Could you check a few things on this model? Use its own coordinates, in mm. A direction names the side the tool comes from. Round coordinates to 2 decimals unless told otherwise and drop trailing zeros. Write each loop counter-clockwise with the first axis right and the second up, starting at its lowest first coordinate (ties: lowest second). Pieces come first, ordered by that corner, then holes. Notation, with made-up numbers: (-14, 67.5) -> (38, 67.5) arc R37 cw to (38, 105.5) -> close; hole circle Ø9 at (70, -34). An arc over 180 degrees is marked (long way). One line per question, with ' | ' between items. Start each with the question number.
1. Imagine slicing it at D-D, the plane y = 33.5. List the corners of the cut face in (x, z) for me.
2. For faces 5 (the flat face through (56.91, -29.28, 0.49)), 6 (the flat face through (-60, -62, 1)), which set-ups out of +Z, -Z, +X, -X, +Y, -Y let a thin tool reach every point of the face, with its end or its side?
3. Imagine slicing it at A-A, the plane y = -37.5. List the corners of the cut face in (x, z) for me, and give its area (3 significant figures).
4. Imagine slicing it at B-B, the plane x = 22. List the corners of the cut face in (y, z) for me, and give its area (3 significant figures).
5. If I drill on line 1 along Y through (x, z) = (52.5, 12.5); line 2 along X through (y, z) = (-51, 13.25); line 3 along Y through (x, z) = (2, 9.25), over which ranges is the centre line in solid material (lowest first)? Write a range as [from, to].
6. Imagine slicing it at C-C, the plane z = 11.25. State how many separate pieces and enclosed holes the cut face has, and give its area (3 significant figures).
7. Thinking about a two-plate mould opening in Y: for faces 1 (the flat face through (-1, 68.5, 12)), 2 (the flat face through (-65.5, -1, 12)), 3 (the flat face through (-63.5, 44, 12)), 4 (the flat face through (32, -66, 12)), which applies, released by +Y, released by -Y, zero draft, split by the parting line, or undercut?
8. For pin 1 Ø6.5 at (x, y) = (59, -17.5) entering from +Z, with a flat end and sliding along its axis, tell me the tip position at first contact or that it passes through.
from build123d import *

# Parameters (mm, degrees)
F0_W     = 131
F0_H     = 137
F1_DEPTH = 24
F2_DEPTH = 1
F3_R     = 2


with BuildPart() as f1:
    # F0 (on Top) → F1 (new body)
    with BuildSketch(Plane.XY):
        Rectangle(F0_W, F0_H)
        Polygon((63.5, -53.262113756), (63.5, -66), (50.5, -66), (13.5, -66), (0.5, -66), (-0.5, -66), (-13.5, -66), (-50.5, -66), (-63.5, -66), (-63.5, -53.262113756), (-63.5, -35.737886244), (-63.5, -23), (-63.5, -21.5), (-63.5, -8.762113756), (-63.5, 8.762113756), (-63.5, 21.5), (-63.5, 23), (-63.5, 35.737886244), (-63.5, 53.262113756), (-63.5, 66), (-50.5, 66), (-13.5, 66), (-0.5, 66), (0.5, 66), (13.5, 66), (50.5, 66), (63.5, 66), (63.5, 53.262113756), (63.5, 35.737886244), (63.5, 23), (63.5, 21.5), (63.5, 8.762113756), (63.5, -8.762113756), (63.5, -21.5), (63.5, -23), (63.5, -35.737886244), align=None, mode=Mode.SUBTRACT)
        Polygon((-0.5, -66), (0.5, -66), (0.5, -53.262113756), (0.5, -35.737886244), (0.5, -23), (0.5, -21.5), (0.5, -8.762113756), (0.5, 8.762113756), (0.5, 21.5), (0.5, 23), (0.5, 35.737886244), (0.5, 53.262113756), (0.5, 66), (-0.5, 66), (-0.5, 53.262113756), (-0.5, 35.737886244), (-0.5, 23), (-0.5, 21.5), (-0.5, 8.762113756), (-0.5, -8.762113756), (-0.5, -21.5), (-0.5, -23), (-0.5, -35.737886244), (-0.5, -53.262113756), align=None)
        Polygon((50.5, 21.5), (63.5, 21.5), (63.5, 23), (50.5, 23), (13.5, 23), (0.5, 23), (0.5, 21.5), (13.5, 21.5), align=None)
        Polygon((-13.5, 21.5), (-0.5, 21.5), (-0.5, 23), (-13.5, 23), (-50.5, 23), (-63.5, 23), (-63.5, 21.5), (-50.5, 21.5), align=None)
        Polygon((-13.5, -23), (-0.5, -23), (-0.5, -21.5), (-13.5, -21.5), (-50.5, -21.5), (-63.5, -21.5), (-63.5, -23), (-50.5, -23), align=None)
        Polygon((50.5, -23), (63.5, -23), (63.5, -21.5), (50.5, -21.5), (13.5, -21.5), (0.5, -21.5), (0.5, -23), (13.5, -23), align=None)
    extrude(amount=F1_DEPTH)

    # F0 (on Top) → F2 (join)
    with BuildSketch(Plane.XY):
        Polygon((-63.5, 66), (-63.5, 53.262113756), (-50.5, 66), align=None)
        Polygon((-63.5, 35.737886244), (-63.5, 23), (-50.5, 23), align=None)
        Polygon((-13.5, 66), (-0.5, 53.262113756), (-0.5, 66), align=None)
        Polygon((-13.5, 23), (-0.5, 23), (-0.5, 35.737886244), align=None)
        Polygon((0.5, 66), (0.5, 53.262113756), (13.5, 66), align=None)
        Polygon((50.5, 66), (63.5, 53.262113756), (63.5, 66), align=None)
        Polygon((50.5, 23), (63.5, 23), (63.5, 35.737886244), align=None)
        Polygon((0.5, 35.737886244), (0.5, 23), (13.5, 23), align=None)
        Polygon((0.5, 21.5), (0.5, 8.762113756), (13.5, 21.5), align=None)
        Polygon((-13.5, 21.5), (-0.5, 8.762113756), (-0.5, 21.5), align=None)
        Polygon((-63.5, 21.5), (-63.5, 8.762113756), (-50.5, 21.5), align=None)
        Polygon((-63.5, -8.762113756), (-63.5, -21.5), (-50.5, -21.5), align=None)
        Polygon((-13.5, -21.5), (-0.5, -21.5), (-0.5, -8.762113756), align=None)
        Polygon((50.5, -21.5), (63.5, -21.5), (63.5, -8.762113756), align=None)
        Polygon((50.5, 21.5), (63.5, 8.762113756), (63.5, 21.5), align=None)
        Polygon((0.5, -8.762113756), (0.5, -21.5), (13.5, -21.5), align=None)
        Polygon((0.5, -23), (0.5, -35.737886244), (13.5, -23), align=None)
        Polygon((-13.5, -23), (-0.5, -35.737886244), (-0.5, -23), align=None)
        Polygon((-63.5, -23), (-63.5, -35.737886244), (-50.5, -23), align=None)
        Polygon((-63.5, -66), (-50.5, -66), (-63.5, -53.262113756), align=None)
        Polygon((-13.5, -66), (-0.5, -66), (-0.5, -53.262113756), align=None)
        Polygon((0.5, -66), (13.5, -66), (0.5, -53.262113756), align=None)
        Polygon((50.5, -23), (63.5, -35.737886244), (63.5, -23), align=None)
        Polygon((50.5, -66), (63.5, -66), (63.5, -53.262113756), align=None)
    extrude(amount=F2_DEPTH)

    # F3
    f3_edges = [f1.edges().sort_by_distance(p)[0] for p in [
        (-65.5, 68.5, 12),
        (65.5, 68.5, 12),
        (-65.5, -68.5, 12),
        (65.5, -68.5, 12),
        (63.5, -23, 12.5),
        (63.5, 66, 12.5),
        (-0.5, 66, 12.5),
        (-0.5, 21.5, 12.5),
        (-0.5, -23, 12.5),
        (63.5, 21.5, 12.5),
        (-63.5, 21.5, 12.5),
        (-63.5, 66, 12.5),
        (-63.5, -23, 12.5),
        (0.5, 66, 12.5),
        (0.5, 21.5, 12.5),
        (0.5, -23, 12.5),
        (-63.5, -66, 12.5),
        (-63.5, -21.5, 12.5),
        (-63.5, 23, 12.5),
        (0.5, 23, 12.5),
        (0.5, -21.5, 12.5),
        (0.5, -66, 12.5),
        (-0.5, -66, 12.5),
        (-0.5, -21.5, 12.5),
        (-0.5, 23, 12.5),
        (63.5, 23, 12.5),
        (63.5, -21.5, 12.5),
        (63.5, -66, 12.5),
    ]]
    fillet(f3_edges, radius=F3_R)


solid = f1.part
Geometry results:
1) outline: (-65.5, 0) -> (-61.22, 0) -> (-61.22, 1) -> (-63.5, 1) -> (-63.5, 24) -> (-65.5, 24) -> close; (-2.78, 0) -> (2.78, 0) -> (2.78, 1) -> (0.5, 1) -> (0.5, 24) -> (-0.5, 24) -> (-0.5, 1) -> (-2.78, 1) -> close; (61.22, 0) -> (65.5, 0) -> (65.5, 24) -> (63.5, 24) -> (63.5, 1) -> (61.22, 1) -> close
2) face 5: +Z, -Z | face 6: +Z
3) outline: (-65.5, 0) -> (-63.5, 0) -> (-63.5, 24) -> (-65.5, 24) -> close; (-0.5, 0) -> (0.5, 0) -> (0.5, 24) -> (-0.5, 24) -> close; (63.5, 0) -> (65.5, 0) -> (65.5, 24) -> (63.5, 24) -> close | area: 120 mm2
4) outline: (-68.5, 0) -> (-66, 0) -> (-66, 24) -> (-68.5, 24) -> close; (-23, 0) -> (-21.5, 0) -> (-21.5, 24) -> (-23, 24) -> close; (21.5, 0) -> (23, 0) -> (23, 24) -> (21.5, 24) -> close; (66, 0) -> (68.5, 0) -> (68.5, 24) -> (66, 24) -> close | area: 192 mm2
5) line 1: y = [-68.5, -66], [-23, -21.5], [21.5, 23], [66, 68.5] | line 2: x = [-65.5, -63.5], [-0.5, 0.5], [63.5, 65.5] | line 3: y = [-68.5, -65.94], [-23.06, -21.44], [21.44, 23.06], [65.94, 68.5]
6) separate pieces: 1 | enclosed holes: 6 | area: 1,710 mm2
7) face 1: released by +Y | face 2: zero draft | face 3: undercut | face 4: undercut
8) pin 1: stops at z = 1
